Build history of the part. All positions in model axes, mm. A direction names the side the tool comes from. Coordinates: 2 decimals unless noted, no trailing zeros. Order: outer loops, then holes, each group sorted by start corner. A loop starts at its lowest first (then second) coordinate and runs counter-clockwise, first axis right, second up. Notation, with made-up numbers: (-12, -29.5) - (5, -29.5) arc R22 ccw to (5, 4.5) - close; hole circle Ø4 at (67, 48). An arc over 180 degrees is marked (long way). Write each question's results on one line, items separated by ' | '.
from build123d import *

# Parameters (mm, degrees)
CYLINDER005_R     = 20
CYLINDER005_DEPTH = 8
SKETCH006_R       = 2.2
SKETCH006_R_2     = 2.75
POCKET004_DEPTH   = 12.001
POCKET005_DEPTH   = 4


with BuildPart() as part:
    # Cylinder005 → Cylinder005 (join)
    with BuildSketch(Plane.XY):
        Circle(CYLINDER005_R)
    extrude(amount=CYLINDER005_DEPTH)

    # Sphere → Sphere (revolve)
    with BuildSketch(Plane(origin=(6, 10.392305, 0), x_dir=(1, 0, 0), z_dir=(0, -1, 0))):
        with BuildLine():
            ThreePointArc((0, -4), (2.828427, -2.828427), (4, 0))
            Line((4, 0), (0, 0))
            Line((0, 0), (0, -4))
        make_face()
    revolve(axis=Axis((6, 10.392305, 0), (0, 0, 1)))

    # Sphere001 → Sphere001 (revolve)
    with BuildSketch(Plane(origin=(6, -10.392305, 0), x_dir=(1, 0, 0), z_dir=(0, -1, 0))):
        with BuildLine():
            ThreePointArc((0, -4), (2.828427, -2.828427), (4, 0))
            Line((4, 0), (0, 0))
            Line((0, 0), (0, -4))
        make_face()
    revolve(axis=Axis((6, -10.392305, 0), (0, 0, 1)))

    # Sketch006 (on DatumPlane) → Pocket004 (cut, through all)
    with BuildSketch(Plane.XY.offset(8)):
        with Locations((-12, 0)):
            Circle(SKETCH006_R)
        with Locations((12, 0)):
            Circle(SKETCH006_R)
        Circle(SKETCH006_R_2)
    extrude(amount=-POCKET004_DEPTH, mode=Mode.SUBTRACT)

    # Sketch063 (on DatumPlane) → Pocket005 (cut)
    with BuildSketch(Plane(origin=(0, 0, 0), x_dir=(1, 0, 0), z_dir=(0, 0, -1))):
        Polygon((-9.892672, -3.65), (-7.785343, 0), (-9.892672, 3.65), (-14.107328, 3.65), (-16.214657, 0), (-14.107328, -3.65), align=None)
        Polygon((14.107328, -3.65), (16.214657, 0), (14.107328, 3.65), (9.892672, 3.65), (7.785343, 0), (9.892672, -3.65), align=None)
    extrude(amount=-POCKET005_DEPTH, mode=Mode.SUBTRACT)


with BuildPart() as part_1:
    # Body022003 placement: moved
    add(part.part.moved(Location((-2.5, 0, 885))))


solid = part_1.part
1. Band-saw the part on A-A on x = -2.5. Give the cut face in (y, z).
Solved:
outline: (-20, 885) - (-2.75, 885) - (-2.75, 893) - (-20, 893) - close; (2.75, 885) - (20, 885) - (20, 893) - (2.75, 893) - close
2. Band-saw the part on D-D on y = 17.5. Give the cut face in (x, z).
Solved:
outline: (-12.18, 885) - (7.18, 885) - (7.18, 893) - (-12.18, 893) - close
3. Drop flat-ended pins along their axis: pin 1 Ø1.5 at (y, z) = (13, 891) entering from -X; pin 2 Ø5 at (x, z) = (6.5, 890) entering from -Y; pin 3 Ø5.5 at (x, y) = (9.5, 0) entering from +Z; pin 4 Ø2 at (x, z) = (9, 887.5) entering from +Y. Give the stop position or say it passes through.
Solved:
pin 1: stops at x = -18.31 | pin 2: stops at y = -18.91 | pin 3: stops at z = 893 | pin 4: stops at y = 17.02
4. Two-plate mould, pull along X, no slides. Class faces 1 (the face through (-3, -4, 885)), 2 (the face through (-15, 3.65, 887)), 3 (the face through (-22.48, 0.88, 888.94)), 4 (the face through (-14, -3.65, 887)): +X half, -X half, draft (parallel to the pull), parting line (faces both ways), or undercut.
Solved:
face 1: draft | face 2: undercut | face 3: parting line | face 4: undercut
5. Band-saw the part on C-C on z = 892.25. Give the cut face in (x, y), then the cut area to 3 significant figures.
Solved:
outline: circle Ø40 at (-2.5, 0); hole circle Ø4.4 at (-14.5, 0); hole circle Ø5.5 at (-2.5, 0); hole circle Ø4.4 at (9.5, 0) | area: 1,200 mm2
6. Tool access for faces 5 (the face through (10, -3.65, 887)), 6 (the face through (-12.468, -0.843, 891.028)): list every direction of +Z, -Z, +X, -X, +Y, -Y with a clear straight run to the whole face (end or side of a thin tool).
Solved:
face 5: -Z | face 6: +Z, -Z
7. Probe line 1 (Y direction, x = -2.5, z = 889.75); line 2 (Z direction, x = -4, y = -3.5); line 3 (Y direction, x = -5, z = 888). List the from-to ranges inside material, lowest first.
Solved:
line 1: y = -20 to -2.75, 2.75 to 20 | line 2: z = 885 to 893 | line 3: y = -19.84 to -1.15, 1.15 to 19.84
8. Band-saw the part on B-B on x = -14.5. Give the cut face in (y, z), then the cut area to 3 significant figures.
Solved:
outline: (-16, 885) - (-3.65, 885) - (-3.65, 889) - (-2.2, 889) - (-2.2, 893) - (-16, 893) - close; (2.2, 889) - (3.65, 889) - (3.65, 885) - (16, 885) - (16, 893) - (2.2, 893) - close | area: 209 mm2
